```python
from build123d import *

# Parameters (mm, degrees)
FILLET1_R           = 2
FILLET2_R           = 6
SCALE1_SCALE        = 0.85
SKETCH4_R           = 10.6
CUT_EXTRUDE2_DEPTH  = 51.23590774
SKETCH9_R           = 2.25
BOSS_EXTRUDE1_DEPTH = 4.25
FILLET4_R           = 3
CUT_EXTRUDE3_DEPTH  = 46.98590774


with BuildPart() as part:
    # Sketch2 → Revolve1 (revolve)
    with BuildSketch(Plane(origin=(0, 0, 0), x_dir=(0, 0, -1), z_dir=(1, 0, 0))):
        Polygon((10.1, 0), (10.1, 6.971067812), (62.23, 59.101067812), (75, 59.101067812), (75, 54.101067812), (64.301067812, 54.101067812), (15.1, 4.9), (20, 0), align=None)
    revolve(axis=Axis((0, 0, 0), (0, 1, 0)))

    # Fillet1
    fillet1_edges = [part.edges().sort_by_distance(p)[0] for p in [
        (0, 4.9, 15.1),
    ]]
    fillet(fillet1_edges, radius=FILLET1_R)

    # Fillet2
    fillet2_edges = [part.edges().sort_by_distance(p)[0] for p in [
        (0, 6.971067812, 10.1),
    ]]
    fillet(fillet2_edges, radius=FILLET2_R)


with BuildPart() as part_1:
    # Scale1: scaled about (0, 40.216103787, 0)
    add(part.part.scale(SCALE1_SCALE).moved(Location((0, 6.032415568, 0))))

    # Sketch4 → Cut-Extrude2 (cut, through all)
    with BuildSketch(Plane.XZ.offset(-6.032415568)):
        Circle(SKETCH4_R)
    extrude(amount=-CUT_EXTRUDE2_DEPTH, mode=Mode.SUBTRACT)

    # Sketch9 → Boss-Extrude1 (add)
    with BuildSketch(Plane.XZ.offset(-52.018323208)):
        with BuildLine():
            Line((-62.154465971, 14.492663996), (-63.814937276, -0.932057036))
            ThreePointArc((-63.814937276, -0.932057036), (-64.336549414, 0.385954164), (-65.60066074, 1.027246064))
            Line((-65.60066074, 1.027246064), (-70.240082919, 1.526679887))
            ThreePointArc((-70.240082919, 1.526679887), (-75.563426885, 8.134403325), (-68.955703447, 13.45774729))
            Line((-68.955703447, 13.45774729), (-64.316281268, 12.958313466))
            ThreePointArc((-64.316281268, 12.958313466), (-62.944644221, 13.315867039), (-62.154465971, 14.492663996))
        make_face()
        with Locations((-69.597893183, 7.492213588)):
            Circle(SKETCH9_R, mode=Mode.SUBTRACT)
        with BuildLine():
            Line((-0.932057036, 63.814937276), (14.492663996, 62.154465971))
            ThreePointArc((14.492663996, 62.154465971), (13.315867039, 62.944644221), (12.958313466, 64.316281268))
            Line((12.958313466, 64.316281268), (13.45774729, 68.955703447))
            ThreePointArc((13.45774729, 68.955703447), (8.134403325, 75.563426885), (1.526679887, 70.240082919))
            Line((1.526679887, 70.240082919), (1.027246064, 65.60066074))
            ThreePointArc((1.027246064, 65.60066074), (0.385954164, 64.336549414), (-0.932057036, 63.814937276))
        make_face()
        with Locations((7.492213588, 69.597893183)):
            Circle(SKETCH9_R, mode=Mode.SUBTRACT)
        with BuildLine():
            Line((63.814937276, 0.932057036), (62.154465971, -14.492663996))
            ThreePointArc((62.154465971, -14.492663996), (62.944644221, -13.315867039), (64.316281268, -12.958313466))
            Line((64.316281268, -12.958313466), (68.955703447, -13.45774729))
            ThreePointArc((68.955703447, -13.45774729), (75.563426885, -8.134403325), (70.240082919, -1.526679887))
            Line((70.240082919, -1.526679887), (65.60066074, -1.027246064))
            ThreePointArc((65.60066074, -1.027246064), (64.336549414, -0.385954164), (63.814937276, 0.932057036))
        make_face()
        with Locations((69.597893183, -7.492213588)):
            Circle(SKETCH9_R, mode=Mode.SUBTRACT)
        with BuildLine():
            Line((-14.492663996, -62.154465971), (0.932057036, -63.814937276))
            ThreePointArc((0.932057036, -63.814937276), (-0.385954164, -64.336549414), (-1.027246064, -65.60066074))
            Line((-1.027246064, -65.60066074), (-1.526679887, -70.240082919))
            ThreePointArc((-1.526679887, -70.240082919), (-8.134403325, -75.563426885), (-13.45774729, -68.955703447))
            Line((-13.45774729, -68.955703447), (-12.958313466, -64.316281268))
            ThreePointArc((-12.958313466, -64.316281268), (-13.315867039, -62.944644221), (-14.492663996, -62.154465971))
        make_face()
        with Locations((-7.492213588, -69.597893183)):
            Circle(SKETCH9_R, mode=Mode.SUBTRACT)
    extrude(amount=-BOSS_EXTRUDE1_DEPTH)

    # Fillet4
    fillet4_edges = [part_1.edges().sort_by_distance(p)[0] for p in [
        (-7.495331881, 13.972823208, 7.495331881),
        (0, 52.018323208, 54.65590764),
    ]]
    fillet(fillet4_edges, radius=FILLET4_R)

    # Sketch11 → Cut-Extrude3 (cut, through all)
    with BuildSketch(Plane.XZ.offset(-52.018323208)):
        with BuildLine():
            Line((-62.220212975, 13.8819162), (-62.154465971, 14.492663996))
            ThreePointArc((-62.154465971, 14.492663996), (-62.944644221, 13.315867039), (-64.316281268, 12.958313466))
            Line((-64.316281268, 12.958313466), (-68.955703447, 13.45774729))
            ThreePointArc((-68.955703447, 13.45774729), (-75.563426885, 8.134403325), (-70.240082919, 1.526679887))
            Line((-70.240082919, 1.526679887), (-65.60066074, 1.027246064))
            ThreePointArc((-65.60066074, 1.027246064), (-64.336549414, 0.385954164), (-63.814937276, -0.932057036))
            Line((-63.814937276, -0.932057036), (-63.749190272, -0.321309239))
            ThreePointArc((-63.749190272, -0.321309239), (-49.643889291, -39.99433405), (-13.8819162, -62.220212975))
            Line((-13.8819162, -62.220212975), (-14.492663996, -62.154465971))
            ThreePointArc((-14.492663996, -62.154465971), (-13.315867039, -62.944644221), (-12.958313466, -64.316281268))
            Line((-12.958313466, -64.316281268), (-13.45774729, -68.955703447))
            ThreePointArc((-13.45774729, -68.955703447), (-8.134403325, -75.563426885), (-1.526679887, -70.240082919))
            Line((-1.526679887, -70.240082919), (-1.027246064, -65.60066074))
            ThreePointArc((-1.027246064, -65.60066074), (-0.385954164, -64.336549414), (0.932057036, -63.814937276))
            Line((0.932057036, -63.814937276), (0.321309239, -63.749190272))
            ThreePointArc((0.321309239, -63.749190272), (39.99433405, -49.643889291), (62.220212975, -13.8819162))
            Line((62.220212975, -13.8819162), (62.154465971, -14.492663996))
            ThreePointArc((62.154465971, -14.492663996), (62.944644221, -13.315867039), (64.316281268, -12.958313466))
            Line((64.316281268, -12.958313466), (68.955703447, -13.45774729))
            ThreePointArc((68.955703447, -13.45774729), (75.563426885, -8.134403325), (70.240082919, -1.526679887))
            Line((70.240082919, -1.526679887), (65.60066074, -1.027246064))
            ThreePointArc((65.60066074, -1.027246064), (64.336549414, -0.385954164), (63.814937276, 0.932057036))
            Line((63.814937276, 0.932057036), (63.749190272, 0.321309239))
            ThreePointArc((63.749190272, 0.321309239), (49.643889291, 39.99433405), (13.8819162, 62.220212975))
            Line((13.8819162, 62.220212975), (14.492663996, 62.154465971))
            ThreePointArc((14.492663996, 62.154465971), (13.315867039, 62.944644221), (12.958313466, 64.316281268))
            Line((12.958313466, 64.316281268), (13.45774729, 68.955703447))
            ThreePointArc((13.45774729, 68.955703447), (8.134403325, 75.563426885), (1.526679887, 70.240082919))
            Line((1.526679887, 70.240082919), (1.027246064, 65.60066074))
            ThreePointArc((1.027246064, 65.60066074), (0.385954164, 64.336549414), (-0.932057036, 63.814937276))
            Line((-0.932057036, 63.814937276), (-0.321309239, 63.749190272))
            ThreePointArc((-0.321309239, 63.749190272), (-39.99433405, 49.643889291), (-62.220212975, 13.8819162))
        make_face()
    extrude(amount=CUT_EXTRUDE3_DEPTH, mode=Mode.SUBTRACT)


solid = part_1.part
```
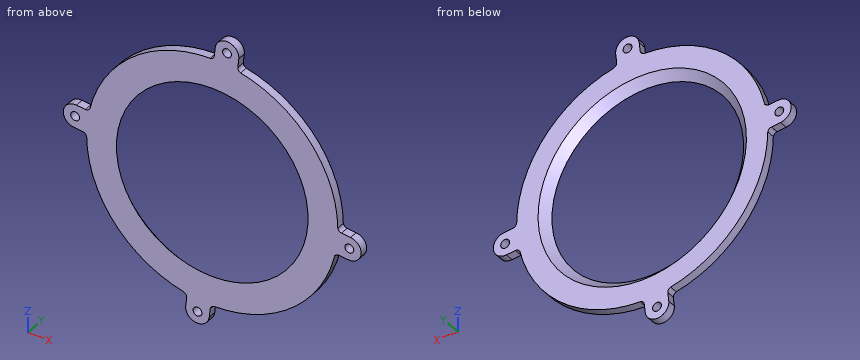
Verification items for the finished model (mm, model axes). Give positions to 0.01 mm unless a question says otherwise; leave off trailing zeros. Loops run counter-clockwise (first coordinate to the right, second up) from the corner with the lowest first, then second, coordinate; pieces in that order, holes last.
1. Go/stop test with flat-tipped pins: pin 1 Ø2 at (y, z) = (55.5, -29) entering from -X; pin 2 Ø2 at (y, z) = (53, -43.5) entering from -X. Record where each tip stops, or that it passes through.
2. Section check C-C, the plane z = -58. Enter the section's corners in (x, y), then the cut area to 3 significant figures.
3. Thickness scan on line 1 (X direction, y = 54.7, z = -7); line 2 (X direction, y = 54.65, z = -6); line 3 (Z direction, x = -9.5, y = 53). Record the ranges inside material, lowest first.
4. Section check A-A, the plane y = 54.7. Count the separate pieces of the cut face and the enclosed holes in it, then the cut area to 3 significant figures.
5. Section check B-B, the plane x = 59.5. Enter the section's corners in (y, z), then the cut area to 3 significant figures.
Geometry says:
1. pin 1: stops at x = -57.27
1. pin 2: stops at x = -47.52
2. outline: (-26.46, 52.02) - (26.46, 52.02) - (26.46, 56.27) - (-26.46, 56.27) - close
2. area: 225 mm2
3. line 1: x = -63.36 to -50.85, 50.85 to 67.4, 71.79 to 75.58
3. line 2: x = -63.47 to -50.92, 50.92 to 67.91, 71.28 to 75.41
3. line 3: z = -75.25 to -70.61, -68.58 to -48.71, 48.71 to 63.04
4. separate pieces: 1
4. enclosed holes: 5
4. area: 4,960 mm2
5. outline: (52.02, -22.89) - (56.27, -22.89) - (56.27, 22.89) - (52.02, 22.89) - close
5. area: 195 mm2
